Build history of the part. All positions in model axes, mm. A direction names the side the tool comes from. Coordinates: 2 decimals unless noted, no trailing zeros. Order: outer loops, then holes, each group sorted by start corner. A loop starts at its lowest first (then second) coordinate and runs counter-clockwise, first axis right, second up. Notation, with made-up numbers: (-9, 63) - (14, 63) arc R20 ccw to (14, 92) - close; hole circle Ø1 at (70.5, 37.25). An arc over 180 degrees is marked (long way). Write each question's results on one line, items separated by ' | '.
from build123d import *

# Parameters (mm, degrees)
SKETCH1_W            = 133
SKETCH1_H            = 133
BOSS_EXTRUDE2_DEPTH  = 136
SKETCH2_W            = 133
SKETCH2_H            = 118
CUT_EXTRUDE1_DEPTH   = 136
BOSS_EXTRUDE3_DEPTH  = 10.5
SKETCH5_W            = 21
SKETCH5_H            = 3
BOSS_EXTRUDE4_DEPTH  = 23.5
SKETCH6_W            = 42
SKETCH6_H            = 17.2
CUT_EXTRUDE2_DEPTH   = 3
BOSS_EXTRUDE5_DEPTH  = 10.5
SKETCH8_W            = 21
SKETCH8_H            = 3
BOSS_EXTRUDE6_DEPTH  = 23.5
SKETCH9_W            = 42
SKETCH9_H            = 17.2
CUT_EXTRUDE3_DEPTH   = 3
SKETCH10_W           = 19.261488562
SKETCH10_H           = 133
BOSS_EXTRUDE7_DEPTH  = 5
SKETCH11_W           = 18.43727499
SKETCH11_H           = 133
BOSS_EXTRUDE8_DEPTH  = 5
SKETCH12_W           = 18.849381776
SKETCH12_H           = 146
BOSS_EXTRUDE9_DEPTH  = 12
SKETCH14_W           = 18.849381776
SKETCH14_H           = 146
BOSS_EXTRUDE10_DEPTH = 12
SKETCH17_R           = 1
CUT_EXTRUDE4_DEPTH   = 222.251553667
SKETCH20_W           = 133.244561713
SKETCH20_H           = 5
CUT_EXTRUDE10_DEPTH  = 19
SKETCH21_W           = 157
SKETCH21_H           = 120.66580897
CUT_EXTRUDE11_DEPTH  = 118
SKETCH22_W           = 186.174267818
SKETCH22_H           = 42.2523161
CUT_EXTRUDE12_DEPTH  = 118
SKETCH23_W           = 12
SKETCH23_H           = 25.33419103
CUT_EXTRUDE13_DEPTH  = 118
SKETCH24_W           = 12
SKETCH24_H           = 25.33419103
CUT_EXTRUDE14_DEPTH  = 118
SKETCH31_R           = 2.5
CUT_EXTRUDE21_DEPTH  = 118
SKETCH32_R           = 2.5
CUT_EXTRUDE22_DEPTH  = 118
SKETCH33_W           = 133
SKETCH33_H           = 5
CUT_EXTRUDE24_DEPTH  = 118
SKETCH34_R           = 2.5
CUT_EXTRUDE25_DEPTH  = 118
SKETCH35_W           = 133
SKETCH35_H           = 133
SKETCH35_W_2         = 86.097023631
SKETCH35_H_2         = 92.508019
CUT_EXTRUDE27_DEPTH  = 10
SKETCH36_R           = 2.5
CUT_EXTRUDE28_DEPTH  = 178
SKETCH37_R           = 2.5
CUT_EXTRUDE29_DEPTH  = 42


with BuildPart() as part:
    # Sketch1 → Boss-Extrude2 (new body)
    with BuildSketch(Plane(origin=(0, 0, 0), x_dir=(1, 0, 0), z_dir=(0, 1, 0))):
        Rectangle(SKETCH1_W, SKETCH1_H)
    extrude(amount=BOSS_EXTRUDE2_DEPTH)

    # Sketch2 → Cut-Extrude1 (cut)
    with BuildSketch(Plane.XY.offset(66.5)):
        with Locations((0, 68)):
            Rectangle(SKETCH2_W, SKETCH2_H)
    extrude(amount=-CUT_EXTRUDE1_DEPTH, mode=Mode.SUBTRACT)


with BuildPart() as cut_extrude1_piece_1:
    # of the separate pieces the step leaves, piece 1, a body of its own (cut_extrude1_pieces)
    add(part.part.solids().sort_by_distance((-66.5, 0, 66.5))[0])

    # Sketch4 → Boss-Extrude3 (add)
    with BuildSketch(Plane(origin=(0, 9, 0), x_dir=(1, 0, 0), z_dir=(0, 1, 0))):
        Polygon((22.75, -22.75), (43.75, -22.75), (46.25, -22.75), (46.25, -20.25), (20.25, -20.25), (20.25, -46.25), (46.25, -46.25), (46.25, -43.75), (43.75, -43.75), (22.75, -43.75), align=None)
        Polygon((22.75, 43.75), (43.75, 43.75), (46.25, 43.75), (46.25, 46.25), (20.25, 46.25), (20.25, 20.25), (46.25, 20.25), (46.25, 22.75), (43.75, 22.75), (22.75, 22.75), align=None)
    extrude(amount=BOSS_EXTRUDE3_DEPTH)

    # Sketch5 → Boss-Extrude4 (add)
    with BuildSketch(Plane(origin=(22.75, 0, 0), x_dir=(0, 0, -1), z_dir=(1, 0, 0))):
        with Locations((-33.25, 18)):
            Rectangle(SKETCH5_W, SKETCH5_H)
        with Locations((33.25, 18)):
            Rectangle(SKETCH5_W, SKETCH5_H)
    extrude(amount=BOSS_EXTRUDE4_DEPTH)

    # Sketch6 → Cut-Extrude2 (cut)
    with BuildSketch(Plane(origin=(0, 19.5, 0), x_dir=(1, 0, 0), z_dir=(0, 1, 0))):
        with Locations((46.25, -33.25)):
            Rectangle(SKETCH6_W, SKETCH6_H)
        with Locations((46.25, 33.25)):
            Rectangle(SKETCH6_W, SKETCH6_H)
    extrude(amount=-CUT_EXTRUDE2_DEPTH, mode=Mode.SUBTRACT)

    # Sketch10 → Boss-Extrude7 (add)
    with BuildSketch(Plane.XZ):
        Rectangle(SKETCH10_W, SKETCH10_H)
    extrude(amount=BOSS_EXTRUDE7_DEPTH)



with BuildPart() as cut_extrude1_piece_2:
    # of the separate pieces the step leaves, piece 2, a body of its own (cut_extrude1_pieces)
    add(part.part.solids().sort_by_distance((66.5, 127, 66.5))[0])

    # Sketch7 → Boss-Extrude5 (add)
    with BuildSketch(Plane.XZ.offset(-127)):
        Polygon((-43.75, 43.75), (-22.75, 43.75), (-22.75, 22.75), (-43.75, 22.75), (-46.25, 22.75), (-46.25, 20.25), (-20.25, 20.25), (-20.25, 46.25), (-46.25, 46.25), (-46.25, 43.75), align=None)
        Polygon((-43.75, -22.75), (-22.75, -22.75), (-22.75, -43.75), (-43.75, -43.75), (-46.25, -43.75), (-46.25, -46.25), (-20.25, -46.25), (-20.25, -20.25), (-46.25, -20.25), (-46.25, -22.75), align=None)
    extrude(amount=BOSS_EXTRUDE5_DEPTH)

    # Sketch8 → Boss-Extrude6 (add)
    with BuildSketch(Plane.ZY.offset(22.75)):
        with Locations((33.25, 118)):
            Rectangle(SKETCH8_W, SKETCH8_H)
        with Locations((-33.25, 118)):
            Rectangle(SKETCH8_W, SKETCH8_H)
    extrude(amount=BOSS_EXTRUDE6_DEPTH)

    # Sketch9 → Cut-Extrude3 (cut)
    with BuildSketch(Plane.XZ.offset(-116.5)):
        with Locations((-46.25, 33.25)):
            Rectangle(SKETCH9_W, SKETCH9_H)
        with Locations((-46.25, -33.25)):
            Rectangle(SKETCH9_W, SKETCH9_H)
    extrude(amount=-CUT_EXTRUDE3_DEPTH, mode=Mode.SUBTRACT)

    # Sketch11 → Boss-Extrude8 (add)
    with BuildSketch(Plane(origin=(0, 136, 0), x_dir=(1, 0, 0), z_dir=(0, 1, 0))):
        Rectangle(SKETCH11_W, SKETCH11_H)
    extrude(amount=BOSS_EXTRUDE8_DEPTH)


with BuildPart() as cut_extrude1_piece_1_1:
    add(cut_extrude1_piece_1.part)

    add(cut_extrude1_piece_2.part)  # Boss-Extrude9 merges Cut-Extrude1 piece 2
    # Sketch12 → Boss-Extrude9 (add)
    with BuildSketch(Plane(origin=(0, 0, -66.5), x_dir=(-1, 0, 0), z_dir=(0, 0, -1))):
        with Locations((-0.206053393, 68)):
            Rectangle(SKETCH12_W, SKETCH12_H)
    extrude(amount=BOSS_EXTRUDE9_DEPTH)

    # Sketch14 → Boss-Extrude10 (add)
    with BuildSketch(Plane.XY.offset(66.5)):
        with Locations((0.206053393, 68)):
            Rectangle(SKETCH14_W, SKETCH14_H)
    extrude(amount=BOSS_EXTRUDE10_DEPTH)

    # Sketch17 → Cut-Extrude4 (cut, through all)
    with BuildSketch(Plane.XY.offset(78.5)):
        with Locations((0.206053393, 68)):
            Circle(SKETCH17_R)
    extrude(amount=-CUT_EXTRUDE4_DEPTH, mode=Mode.SUBTRACT)

    # Sketch20 → Cut-Extrude10 (cut)
    with BuildSketch(Plane.ZY.offset(9.218637495)):
        with Locations((0.122280857, 138.5)):
            Rectangle(SKETCH20_W, SKETCH20_H)
    extrude(amount=-CUT_EXTRUDE10_DEPTH, mode=Mode.SUBTRACT)

    # Sketch21 → Cut-Extrude11 (cut)
    with BuildSketch(Plane.ZY.offset(9.218637495)):
        with Locations((0, 80.667095515)):
            Rectangle(SKETCH21_W, SKETCH21_H)
    extrude(amount=-CUT_EXTRUDE11_DEPTH, mode=Mode.SUBTRACT)


with BuildPart() as cut_extrude11_piece_1:
    # of the separate pieces the step leaves, piece 1, a body of its own (cut_extrude11_pieces)
    add(cut_extrude1_piece_1_1.part.solids().sort_by_distance((9.630744281, 20.33419103, 66.5))[0])

    # Sketch23 → Cut-Extrude13 (cut)
    with BuildSketch(Plane.ZY.offset(9.218637495)):
        with Locations((-72.5, 7.667095515)):
            Rectangle(SKETCH23_W, SKETCH23_H)
    extrude(amount=-CUT_EXTRUDE13_DEPTH, mode=Mode.SUBTRACT)

    # Sketch24 → Cut-Extrude14 (cut)
    with BuildSketch(Plane.ZY.offset(9.218637495)):
        with Locations((72.5, 7.667095515)):
            Rectangle(SKETCH24_W, SKETCH24_H)
    extrude(amount=-CUT_EXTRUDE14_DEPTH, mode=Mode.SUBTRACT)

    # Sketch31 → Cut-Extrude21 (cut)
    with BuildSketch(Plane.XZ.offset(5)):
        with Locations(Location((0, 59.499471122, 0), (0, 0, 270))):
            Circle(SKETCH31_R)
    extrude(amount=-CUT_EXTRUDE21_DEPTH, mode=Mode.SUBTRACT)

    # Sketch32 → Cut-Extrude22 (cut)
    with BuildSketch(Plane.XZ.offset(5)):
        with Locations(Location((0, -59.159797643, 0), (0, 0, 270))):
            Circle(SKETCH32_R)
    extrude(amount=-CUT_EXTRUDE22_DEPTH, mode=Mode.SUBTRACT)

    # Sketch33 → Cut-Extrude24 (cut)
    with BuildSketch(Plane.ZY.offset(9.630744281)):
        with Locations((0, -2.5)):
            Rectangle(SKETCH33_W, SKETCH33_H)
    extrude(amount=-CUT_EXTRUDE24_DEPTH, mode=Mode.SUBTRACT)

    # Sketch34 → Cut-Extrude25 (cut)
    with BuildSketch(Plane(origin=(0, 9, 0), x_dir=(1, 0, 0), z_dir=(0, 1, 0))):
        with Locations(Location((0, 0, 0), (0, 0, 270))):
            Circle(SKETCH34_R)
    extrude(amount=-CUT_EXTRUDE25_DEPTH, mode=Mode.SUBTRACT)

    # Sketch35 → Cut-Extrude27 (cut)
    with BuildSketch(Plane(origin=(0, 9, 0), x_dir=(1, 0, 0), z_dir=(0, 1, 0))):
        Rectangle(SKETCH35_W, SKETCH35_H)
        with Locations((3.201488185, -0.0040095)):
            Rectangle(SKETCH35_W_2, SKETCH35_H_2, mode=Mode.SUBTRACT)
    extrude(amount=-CUT_EXTRUDE27_DEPTH, mode=Mode.SUBTRACT)

    # Sketch36 → Cut-Extrude28 (cut)
    with BuildSketch(Plane(origin=(0, 9, 0), x_dir=(1, 0, 0), z_dir=(0, 1, 0))):
        with Locations(Location((0, 37.126366322, 0), (0, 0, 270))):
            Circle(SKETCH36_R)
    extrude(amount=-CUT_EXTRUDE28_DEPTH, mode=Mode.SUBTRACT)

    # Sketch37 → Cut-Extrude29 (cut)
    with BuildSketch(Plane(origin=(0, 9, 0), x_dir=(1, 0, 0), z_dir=(0, 1, 0))):
        with Locations(Location((0, -34.245307912, 0), (0, 0, 270))):
            Circle(SKETCH37_R)
    extrude(amount=-CUT_EXTRUDE29_DEPTH, mode=Mode.SUBTRACT)


with BuildPart() as cut_extrude11_piece_2:
    # of the separate pieces the step leaves, piece 2, a body of its own (cut_extrude11_pieces)
    add(cut_extrude1_piece_1_1.part.solids().sort_by_distance((-9.218637495, 127, 66.5))[0])

    # Sketch22 → Cut-Extrude12 (cut)
    with BuildSketch(Plane.ZY.offset(66.5)):
        with Locations((20.706035589, 120.536042421)):
            Rectangle(SKETCH22_W, SKETCH22_H)
    extrude(amount=-CUT_EXTRUDE12_DEPTH, mode=Mode.SUBTRACT)


solid = cut_extrude11_piece_1.part
1. Tool access for faces 1 (the face through (33, 14, -20.25)), 2 (the face through (20.25, 14, -33)), 3 (the face through (25.25, 18, 33)), 4 (the face through (22.75, 13, 33)): list every direction of +Z, -Z, +X, -X, +Y, -Y with a clear straight run to the whole face (end or side of a thin tool).
Solved:
face 1: +X, -X, +Y | face 2: +Z, -Z, -X, +Y | face 3: +X, +Y | face 4: +X
2. Band-saw the part on B-B on x = 0. Give the cut face in (y, z), then the cut area to 3 significant figures.
Solved:
outline: (0, -46.25) - (9, -46.25) - (9, -39.63) - (0, -39.63) - close; (0, -34.63) - (9, -34.63) - (9, -2.5) - (0, -2.5) - close; (0, 2.5) - (9, 2.5) - (9, 31.75) - (0, 31.75) - close; (0, 36.75) - (9, 36.75) - (9, 46.26) - (0, 46.26) - close | area: 698 mm2
3. Drop flat-ended pins along their axis: pin 1 Ø6.5 at (x, z) = (40, 38) entering from +Y; pin 2 Ø3 at (x, y) = (27, 15) entering from +Z; pin 3 Ø3 at (y, z) = (14.5, -31) entering from -X. Give the stop position or say it passes through.
Solved:
pin 1: stops at y = 9 | pin 2: stops at z = 46.25 | pin 3: stops at x = 20.25
4. Probe line 1 (Y direction, x = 38, z = 23); line 2 (Z direction, x = 21, y = 18.5); line 3 (X direction, y = 10.25, z = -29.5). List the from-to ranges inside material, lowest first.
Solved:
line 1: y = 0 to 9, 16.5 to 19.5 | line 2: z = -46.25 to -20.25, 20.25 to 46.25 | line 3: x = 20.25 to 22.75
5. Band-saw the part on D-D on z = 30. Give the cut face in (x, y).
Solved:
outline: (-39.85, 0) - (46.25, 0) - (46.25, 9) - (22.75, 9) - (22.75, 16.5) - (25.25, 16.5) - (25.25, 19.5) - (20.25, 19.5) - (20.25, 9) - (-39.85, 9) - close
6. Band-saw the part on A-A on z = 0. Give the cut face in (x, y).
Solved:
outline: (-39.85, 0) - (-2.5, 0) - (-2.5, 9) - (-39.85, 9) - close; (2.5, 0) - (46.25, 0) - (46.25, 9) - (2.5, 9) - close
7. Band-saw the part on C-C on y = 11.75. Give the cut face in (x, z).
Solved:
outline: (20.25, -46.25) - (46.25, -46.25) - (46.25, -43.75) - (22.75, -43.75) - (22.75, -22.75) - (46.25, -22.75) - (46.25, -20.25) - (20.25, -20.25) - close; (20.25, 20.25) - (46.25, 20.25) - (46.25, 22.75) - (22.75, 22.75) - (22.75, 43.75) - (46.25, 43.75) - (46.25, 46.25) - (20.25, 46.25) - close
8. Two-plate mould, pull along Z, no slides. Class faces 5 (the face through (36, 18, 41.85)), 6 (the face through (20.25, 14, 33)), 7 (the face through (3, 5, 46.258)): +Z half, -Z half, draft (parallel to the pull), parting line (faces both ways), or undercut.
Solved:
face 5: undercut | face 6: draft | face 7: +Z half
